Work out the finished part from the listing and answer in its coordinate system (mm). Give positions to 0.01 mm unless a question says otherwise; leave off trailing zeros. Order: outer loops, then holes, each group sorted by start corner. A loop starts at its lowest first (then second) coordinate and runs counter-clockwise, first axis right, second up. Notation, with made-up numbers: (47, 8) - (96, 8) arc R26 ccw to (96, 41) - close; hole circle Ø1 at (64.25, -3.75). An arc over 180 degrees is marked (long way). Write each question's results on one line, items separated by ' | '.
Autodesk Inventor part; units mm, degrees
ref_plane "YZ Plane" through (0, 0, 0) normal (1, 0, 0) x (0, 1, 0)
ref_plane "XZ Plane" through (0, 0, 0) normal (0, 1, 0) x (-1, 0, 0)
ref_plane "XY Plane" through (0, 0, 0) normal (0, 0, 1) x (1, 0, 0)
sketch "Sketch1" plane through (0, 0, 0) normal (0, 1, 0) x (-1, 0, 0)
  circle A0 centre (0, 0) radius 2.5
  dimension "d0" = 5
extrude "Extrusion1" add sketch "Sketch1" along normal blind 128
sketch "Sketch2" plane through (0, 0, 0) normal (1, 0, 0) x (0, 1, 0)
  circle A0 centre (4.6563, 0) radius 2
  point P0 (0, 0)
  dimension "d3" = 4
extrude "Extrusion2" add sketch "Sketch2" along normal blind 80 and the other way blind 3
properties part number "AssemblyAnalysis"
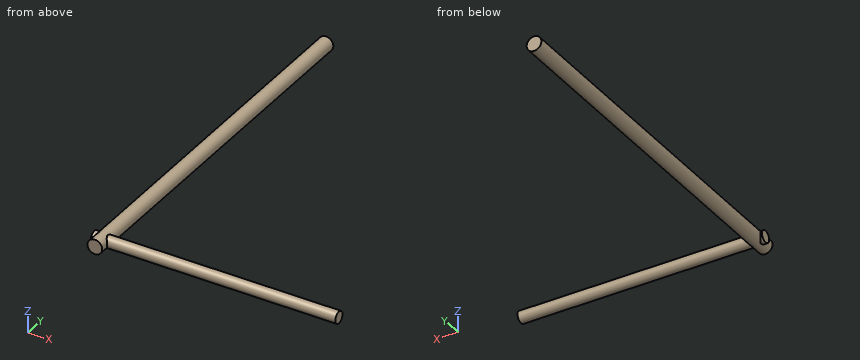
1. A cutting plane is placed at C-C, the plane x = 47.5. Write down the section's boundary in (y, z), then the cut area to 3 significant figures.
Answer list:
outline: circle Ø4 at (4.66, 0) | area: 12.6 mm^2
2. A cutting plane is placed at A-A, the plane z = 0. Write down the section's boundary in (x, y), then the cut area to 3 significant figures.
Answer list:
outline: (-3, 2.66) - (-2.5, 2.66) - (-2.5, 0) - (2.5, 0) - (2.5, 2.66) - (80, 2.66) - (80, 6.66) - (2.5, 6.66) - (2.5, 128) - (-2.5, 128) - (-2.5, 6.66) - (-3, 6.66) - close | area: 952 mm^2
3. Given P1, Ø1.5, axis at x = 11, z = -2, coming from the +Y side; P2, Ø2, axis at y = 110, z = 0.5, coming from the -X side; P3, Ø1.5, axis at y = 25, z = 0.5, coming from the +X side, each flat-ended and moving along its own axis, determine where each tip first touches the part or whether it passes through.
Answer list:
P1: y = 6.22 | P2: x = -2.5 | P3: x = 2.5
4. Straight lines are drawn through the part: line 1 (Z direction, x = 1.5, y = 69); line 2 (Y direction, x = 61, z = -0.3); line 3 (X direction, y = 86, z = 0). For each, find the intervals that lie inside material, in ascending order. Write a range as [from, to].
Answer list:
line 1: [-2, 2] | line 2: [2.68, 6.63] | line 3: [-2.5, 2.5]
5. A cutting plane is placed at B-B, the plane y = 73.5. Write down the section's boundary in (x, z), then the cut area to 3 significant figures.
Answer list:
outline: circle Ø5 at (0, 0) | area: 19.6 mm^2
